from build123d import *

# Parameters (mm, degrees)
F0_R     = 3.3
F0_R_2   = 2.5
F1_DEPTH = 5


with BuildPart() as f1:
    # F0 (on Right) → F1 (new body)
    with BuildSketch(Plane.YZ):
        with BuildLine():
            ThreePointArc((21.963381, 10.731182), (21.963038, 10.725257), (21.962693, 10.719332))
            ThreePointArc((21.962693, 10.719332), (22.073674, 10.724516), (22.184469, 10.732781))
            ThreePointArc((22.184469, 10.732781), (22.073925, 10.73196), (21.963381, 10.731182))
        make_face()
        with BuildLine():
            ThreePointArc((21.462557, 10.734239), (21.646861, 10.721449), (21.831558, 10.717182))
            Line((21.831558, 10.717182), (21.579958, 10.728812))
            Line((21.579958, 10.728812), (21.462557, 10.734239))
        make_face()
        with BuildLine():
            ThreePointArc((21.831558, 10.717182), (21.897134, 10.71772), (21.962693, 10.719332))
            ThreePointArc((21.962693, 10.719332), (21.963038, 10.725257), (21.963381, 10.731182))
            ThreePointArc((21.963381, 10.731182), (21.77167, 10.729933), (21.579958, 10.728812))
            Line((21.579958, 10.728812), (21.831558, 10.717182))
        make_face()
        with BuildLine():
            ThreePointArc((22.184469, 10.732781), (22.073674, 10.724516), (21.962693, 10.719332))
            ThreePointArc((21.962693, 10.719332), (21.897134, 10.71772), (21.831558, 10.717182))
            ThreePointArc((21.831558, 10.717182), (21.646861, 10.721449), (21.462557, 10.734239))
            Line((21.462557, 10.734239), (-2.061471, 11.821605))
            ThreePointArc((-2.061471, 11.821605), (-7.98857, -8.954482), (11.979296, -0.704597))
            ThreePointArc((11.979296, -0.704597), (12.007482, -0.482238), (12.065266, -0.265676))
            Line((12.065266, -0.265676), (12.582355, 3.74023))
            ThreePointArc((12.582355, 3.74023), (13.245307, 4.986202), (14.565898, 5.484191))
            Line((14.565898, 5.484191), (34.746018, 5.484191))
            ThreePointArc((34.746018, 5.484191), (35.491172, 5.340193), (36.129026, 4.928936))
            Line((36.129026, 4.928936), (39.796153, 1.418513))
            ThreePointArc((39.796153, 1.418513), (40.434006, 1.007255), (41.179161, 0.863258))
            Line((41.179161, 0.863258), (51.156007, 0.863258))
            ThreePointArc((51.156007, 0.863258), (51.304636, 0.868788), (51.452444, 0.885349))
            Line((51.452444, 0.885349), (68.043756, 3.371954))
            ThreePointArc((68.043756, 3.371954), (69.216393, 3.862727), (70.01494, 4.851797))
            Line((70.01494, 4.851797), (71.526809, 8.134342))
            ThreePointArc((71.526809, 8.134342), (72.064516, 8.835349), (72.851775, 9.2363))
            Line((72.851775, 9.2363), (93.001659, 14.346079))
            ThreePointArc((93.001659, 14.346079), (93.95316, 14.353851), (94.800564, 13.921045))
            Line((94.800564, 13.921045), (100.556748, 8.949467))
            ThreePointArc((100.556748, 8.949467), (101.307844, 8.541964), (102.160474, 8.485161))
            Line((102.160474, 8.485161), (118.293149, 10.903028))
            ThreePointArc((118.293149, 10.903028), (119.516973, 11.581397), (119.996656, 12.895869))
            ThreePointArc((119.996656, 12.895869), (119.811332, 18.726411), (119.342875, 24.541058))
            ThreePointArc((119.342875, 24.541058), (118.50203, 25.969609), (116.872434, 26.273241))
            Line((116.872434, 26.273241), (78.344445, 16.718787))
            ThreePointArc((78.344445, 16.718787), (50.412085, 12.340754), (22.184469, 10.732781))
        make_face()
        with BuildLine():
            ThreePointArc((-9.809251, -1.943858), (-9.601109, -1.114802), (-8.828326, -0.749472))
            Line((-8.828326, -0.749472), (-6.260139, -0.749472))
            ThreePointArc((-6.260139, -0.749472), (-5.655635, -0.95287), (-5.297041, -1.480323))
            ThreePointArc((-5.297041, -1.480323), (-3.88922, -3.888954), (-1.480686, -5.29694))
            ThreePointArc((-1.480686, -5.29694), (-0.95327, -5.655553), (-0.749901, -6.260046))
            Line((-0.749901, -6.260046), (-0.749969, -8.828254))
            ThreePointArc((-0.749969, -8.828254), (-1.11533, -9.601037), (-1.94441, -9.809142))
            ThreePointArc((-1.94441, -9.809142), (-7.071267, -7.070869), (-9.809251, -1.943858))
        make_face(mode=Mode.SUBTRACT)
        with BuildLine():
            ThreePointArc((9.809251, -1.943858), (7.071068, -7.071068), (1.943858, -9.809251))
            ThreePointArc((1.943858, -9.809251), (1.114802, -9.601109), (0.749472, -8.828326))
            Line((0.749472, -8.828326), (0.749472, -6.260139))
            ThreePointArc((0.749472, -6.260139), (0.95287, -5.655635), (1.480323, -5.297041))
            ThreePointArc((1.480323, -5.297041), (3.889087, -3.889087), (5.297041, -1.480323))
            ThreePointArc((5.297041, -1.480323), (5.655635, -0.95287), (6.260139, -0.749472))
            Line((6.260139, -0.749472), (8.828326, -0.749472))
            ThreePointArc((8.828326, -0.749472), (9.601109, -1.114802), (9.809251, -1.943858))
        make_face(mode=Mode.SUBTRACT)
        Circle(F0_R, mode=Mode.SUBTRACT)
        with BuildLine():
            Line((-6.260139, 0.749472), (-8.828326, 0.749472))
            ThreePointArc((-8.828326, 0.749472), (-9.601109, 1.114802), (-9.809251, 1.943858))
            ThreePointArc((-9.809251, 1.943858), (-7.07108, 7.071056), (-1.943892, 9.809245))
            ThreePointArc((-1.943892, 9.809245), (-1.114823, 9.601096), (-0.749503, 8.828294))
            Line((-0.749503, 8.828294), (-0.749571, 6.260086))
            ThreePointArc((-0.749571, 6.260086), (-0.952972, 5.655604), (-1.480406, 5.297018))
            ThreePointArc((-1.480406, 5.297018), (-3.889118, 3.889057), (-5.297041, 1.480323))
            ThreePointArc((-5.297041, 1.480323), (-5.655635, 0.95287), (-6.260139, 0.749472))
        make_face(mode=Mode.SUBTRACT)
        with BuildLine():
            Line((0.749472, 6.260139), (0.749472, 8.828326))
            ThreePointArc((0.749472, 8.828326), (1.114802, 9.601109), (1.943858, 9.809251))
            ThreePointArc((1.943858, 9.809251), (7.071068, 7.071068), (9.809251, 1.943858))
            ThreePointArc((9.809251, 1.943858), (9.601109, 1.114802), (8.828326, 0.749472))
            Line((8.828326, 0.749472), (6.260139, 0.749472))
            ThreePointArc((6.260139, 0.749472), (5.655635, 0.95287), (5.297041, 1.480323))
            ThreePointArc((5.297041, 1.480323), (3.889087, 3.889087), (1.480323, 5.297041))
            ThreePointArc((1.480323, 5.297041), (0.95287, 5.655635), (0.749472, 6.260139))
        make_face(mode=Mode.SUBTRACT)
        with BuildLine():
            ThreePointArc((46.19369, 9.799431), (47.077203, 9.35514), (47.146779, 8.368656))
            ThreePointArc((47.146779, 8.368656), (46.896258, 6.054576), (48.152498, 4.095088))
            Line((48.152498, 4.095088), (47.670785, 3.330302))
            ThreePointArc((47.670785, 3.330302), (47.307883, 2.98777), (46.824642, 2.863258))
            Line((46.824642, 2.863258), (41.585667, 2.863258))
            ThreePointArc((41.585667, 2.863258), (41.209086, 2.936874), (40.88795, 3.146884))
            Line((40.88795, 3.146884), (36.305408, 7.610078))
            ThreePointArc((36.305408, 7.610078), (36.069285, 8.684144), (36.96252, 9.325627))
            Line((36.96252, 9.325627), (46.19369, 9.799431))
        make_face(mode=Mode.SUBTRACT)
        with Locations((50.303187, 6.856344)):
            Circle(F0_R_2, mode=Mode.SUBTRACT)
        with BuildLine():
            Line((67.125234, 5.256629), (55.291258, 3.483024))
            ThreePointArc((55.291258, 3.483024), (54.838264, 3.519554), (54.448218, 3.752796))
            Line((54.448218, 3.752796), (53.764933, 4.412935))
            ThreePointArc((53.764933, 4.412935), (53.480633, 4.92884), (53.536072, 5.515279))
            ThreePointArc((53.536072, 5.515279), (53.772295, 7.320339), (53.070006, 8.999872))
            ThreePointArc((53.070006, 8.999872), (52.93551, 9.992236), (53.72869, 10.60358))
            Line((53.72869, 10.60358), (69.352887, 12.681545))
            ThreePointArc((69.352887, 12.681545), (70.289379, 12.284015), (70.393014, 11.271934))
            Line((70.393014, 11.271934), (67.885307, 5.827244))
            ThreePointArc((67.885307, 5.827244), (67.577394, 5.445867), (67.125234, 5.256629))
        make_face(mode=Mode.SUBTRACT)
        with BuildLine():
            ThreePointArc((105.708219, 21.280173), (106.727909, 20.958857), (106.874517, 19.89984))
            ThreePointArc((106.874517, 19.89984), (106.863277, 15.788601), (109.9374, 13.058734))
            ThreePointArc((109.9374, 13.058734), (110.062622, 12.958027), (110.08565, 12.798992))
            Line((110.08565, 12.798992), (109.998683, 12.429304))
            ThreePointArc((109.998683, 12.429304), (109.708097, 11.927734), (109.188068, 11.671643))
            Line((109.188068, 11.671643), (103.109307, 10.668558))
            ThreePointArc((103.109307, 10.668558), (102.696959, 10.686849), (102.327124, 10.870116))
            Line((102.327124, 10.870116), (95.85372, 15.977033))
            ThreePointArc((95.85372, 15.977033), (95.561116, 16.351886), (95.474738, 16.819509))
            Line((95.474738, 16.819509), (95.535401, 17.875044))
            ThreePointArc((95.535401, 17.875044), (95.759171, 18.450139), (96.277906, 18.784384))
            Line((96.277906, 18.784384), (105.708219, 21.280173))
        make_face(mode=Mode.SUBTRACT)
        with Locations((111.426774, 17.831758)):
            Circle(F0_R_2, mode=Mode.SUBTRACT)
    extrude(amount=F1_DEPTH)


solid = f1.part
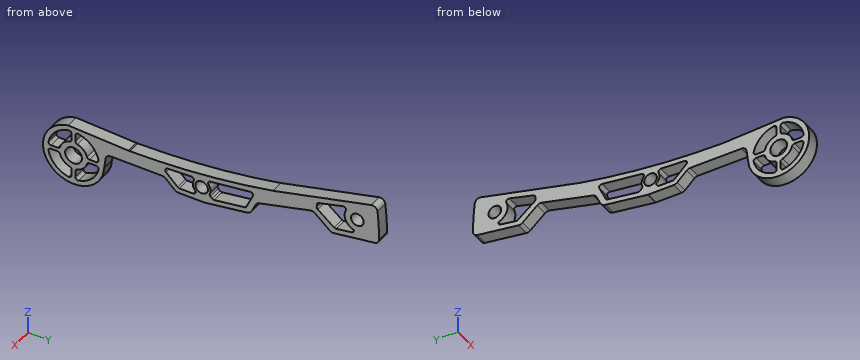
Geometry: final body of the model. Coordinates: model frame, mm. Coordinates: 2 decimals unless noted, no trailing zeros. Return JSON: item names as keys, results as strings.
Item 1: Section query A-A (x = 4.2). Count the separate pieces of the cut face and the enclosed holes in it, and give its area (3 significant figures).
Completed:
{"separate pieces": "1", "enclosed holes": "10", "area": "948 mm2"}
Item 2: Line query: L1, parallel to Y at x = 0.85, z = -4; L2, parallel to Z at x = 2.5, y = 5; L3, parallel to Z at x = 2.75, y = 1. Output: solid intervals per line, ascending.
Completed:
{"L1": "y = -11.31 to -9.17, -3.77 to 3.77, 9.17 to 11.31", "L2": "z = -10.91 to -8.66, -2.29 to 2.29, 8.66 to 11.5", "L3": "z = -11.96 to -9.49, -5.6 to -3.14, 3.14 to 5.6, 9.49 to 11.68"}
Item 3: Pin query (flat end, axial travel): pin 1 Ø3 at (y, z) = (50.3, 6.86) entering from -X; pin 2 Ø1.3 at (x, y) = (3, -7.5) entering from +Z; pin 3 Ø1.5 at (x, y) = (3.5, 47) entering from -Z; pin 4 Ø1.3 at (x, z) = (2.5, -8) entering from -Y. Return the tip coordinate at first contact, or that it passes through.
Completed:
{"pin 1": "passes through", "pin 2": "stops at z = 9.85", "pin 3": "stops at z = 0.86", "pin 4": "stops at y = -9.49"}
